Design review of the part built by this model. Coordinates are the model's own, in mm. Coordinates: 2 decimals unless noted, no trailing zeros. Write each loop counter-clockwise with the first axis right and the second up, starting at its lowest first coordinate (ties: lowest second). Pieces come first, ordered by that corner, then holes. Notation, with made-up numbers: (46, 81) -> (83, 81) arc R27 ccw to (83, 100) -> close; hole circle Ø1 at (-33, 21.5). An arc over 180 degrees is marked (long way). One line per question, with ' | ' between items. Start each with the question number.
Q1. For P1, Ø3, axis at y = 64, z = 12.5, coming from the +X side; P2, Ø1, axis at x = -16, z = -18, coming from the +Y side; P3, Ø10, axis at y = 58.5, z = -1, coming from the +X side, all flat-tipped, find the tip position at first contact; note any pin that passes through.
Q2. Add section B-B on y = 64. State the section outline as (x, z) points.
Q3. Add section A-A on z = 21.5. State the section outline as (x, y) points, and give its area (3 significant figures).
Q4. Add section C-C on x = -22.5. State the section outline as (y, z) points, and give its area (4 significant figures).
Q5. Wall thickness on probe 1 along Y at (x, z) = (-20, -19); probe 2 along Y at (x, z) = (-5.5, -7.5); probe 3 along X at (y, z) = (74, -0.5): over which ranges is each line inside the solid? List them lowest first.
Autodesk Fusion 360 part; units mm, degrees
sketch "Sketch1" plane through (0, 0, 0) normal (0, 0, 1) x (1, 0, 0)
  line L0 (0, 0) -> (-75, 0)
  line L1 (-75, 0) -> (-75, 80)
  line L2 (-75, 80) -> (-30, 80)
  line L3 (-30, 80) -> (0, 50)
  line L4 (0, 50) -> (0, 0)
  dimension "d1" = 75
  dimension "d2" = 80
  dimension "d3" = 135
  dimension "d4" = 50
extrude "Extrude1" add sketch "Sketch1" along normal mid plane 50
Output values:
1) P1: stops at x = -12.5 | P2: stops at y = 66.5 | P3: stops at x = -3.5
2) outline: (-75, -25) -> (-14, -25) -> (-14, 25) -> (-75, 25) -> close
3) outline: (-75, 0) -> (0, 0) -> (0, 50) -> (-30, 80) -> (-75, 80) -> close | area: 5,550 mm2
4) outline: (0, -25) -> (72.5, -25) -> (72.5, 25) -> (0, 25) -> close | area: 3,625 mm2
5) probe 1: y = 0 to 70 | probe 2: y = 0 to 55.5 | probe 3: x = -75 to -24
